Build history of the part. All positions in model axes, mm. Give positions to 0.01 mm unless a question says otherwise; leave off trailing zeros. Loops run counter-clockwise (first coordinate to the right, second up) from the corner with the lowest first, then second, coordinate; pieces in that order, holes last. Notation, with made-up numbers: M 60,31.5 L 104,31.5 A14 cw 104,50.5 Z; hole C 78.5,-12 d4. An arc over 180 degrees is marked long. Answer as a JSON object with one key per item and string values. Group by question number.
1. Slice it at C-C (x = 31.5). List the corners of the cut face in (y, z).
2. Drill centre lines: line 1 along X through (y, z) = (1.9, -36); line 2 along X through (y, z) = (2.45, -12); line 3 along Z through (x, y) = (173.5, 2.35). Where is each one in solid material? Low to high. Write a range as [from, to].
3. Drop flat-ended pins along their axis: pin 1 Ø2.5 at (y, z) = (2, -9) entering from -X; pin 2 Ø1.5 at (y, z) = (1.5, -28.5) entering from +X; pin 3 Ø2.5 at (x, y) = (30, 3) entering from -Z. Give the stop position or say it passes through.
4. Slice it at A-A (z = -28.5). List the corners of the cut face in (x, y), then the cut area to 3 significant figures.
5. Slice it at B-B (y = 2.8). Give the number of separate pieces and of enclosed holes in the cut face, then the cut area to 3 significant figures.
from build123d import *

# Parameters (mm, degrees)
SKETCH_1_W      = 5
SKETCH_1_H      = 10
EXTRUDE_1_DEPTH = 5


with BuildPart() as part:
    # 草图1 → 凸台-拉伸1 (new body)
    with BuildSketch(Plane(origin=(0, 0, 0), x_dir=(1, 0, 0), z_dir=(0, 1, 0))):
        Polygon((0, 0), (200, 0), (200, 5), (195, 5), (195, 15), (200, 15), (200, 25), (195, 25), (195, 35), (200, 35), (200, 40), (175, 40), (175, 35), (165, 35), (165, 40), (110, 40), (110, 35), (90, 35), (90, 40), (35, 40), (35, 35), (25, 35), (25, 40), (0, 40), (-35, 40), (-35, 35), (-30, 35), (-30, 25), (-35, 25), (-35, 15), (-30, 15), (-30, 5), (-35, 5), (-35, 0), align=None)
        with Locations((2.5, 30)):
            Rectangle(SKETCH_1_W, SKETCH_1_H, mode=Mode.SUBTRACT)
        with Locations((2.5, 10)):
            Rectangle(SKETCH_1_W, SKETCH_1_H, mode=Mode.SUBTRACT)
    extrude(amount=EXTRUDE_1_DEPTH)


solid = part.part
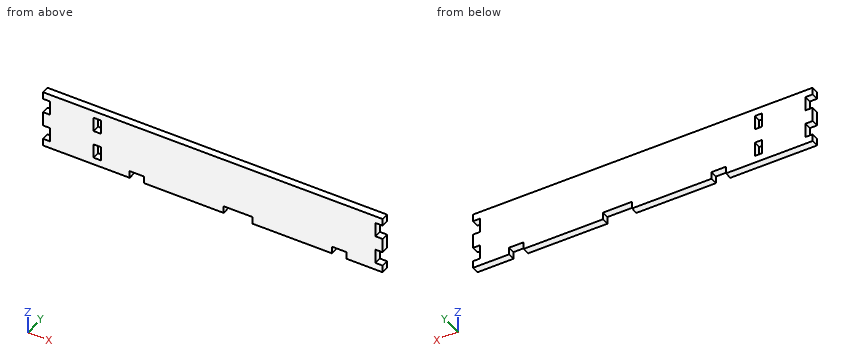
Established:
{
 "1": {"outline": "M 0,-35 L 5,-35 L 5,0 L 0,0 Z"},
 "2": {"line 1": "x = [-35, 25], [35, 90], [110, 165], [175, 200]", "line 2": "x = [-30, 0], [5, 195]", "line 3": "z = [-35, 0]"},
 "3": {"pin 1": "stops at x = -30", "pin 2": "stops at x = 195", "pin 3": "stops at z = -35"},
 "4": {"outline": "M -30,0 L 0,0 L 0,5 L -30,5 Z; M 5,0 L 195,0 L 195,5 L 5,5 Z", "area": "1,100 mm^2"},
 "5": {"separate pieces": "1", "enclosed holes": "2", "area": "8,900 mm^2"}
}
